Work out the finished part from the listing and answer in its coordinate system (mm). Face numbers are marked on the shaded views. Round coordinates to 2 decimals unless told otherwise and drop trailing zeros. Order: outer loops, then holes, each group sorted by start corner. A loop starts at its lowest first (then second) coordinate and runs counter-clockwise, first axis right, second up. Notation, with made-up numbers: (-37, -39) -> (-26, -39) arc R25 cw to (-26, -13) -> close; hole circle Ø9 at (85, 26). An arc over 180 degrees is marked (long way). Use one line per item in the form item = value.
```python
from build123d import *

# Parameters (mm, degrees)
SKETCH1_W           = 88.9
SKETCH1_H           = 38.1
BOSS_EXTRUDE1_DEPTH = 6.35
CUT_EXTRUDE2_DEPTH  = 6.35


with BuildPart() as part:
    # Sketch1 → Boss-Extrude1 (new body)
    with BuildSketch(Plane.YZ):
        with Locations((44.45, 19.05)):
            Rectangle(SKETCH1_W, SKETCH1_H)
    extrude(amount=BOSS_EXTRUDE1_DEPTH)

    # Sketch2 → Cut-Extrude2 (cut)
    with BuildSketch(Plane.YZ.offset(6.35)):
        with BuildLine():
            Line((31.75, 38.1), (57.15, 38.1))
            ThreePointArc((57.15, 38.1), (44.45, 30.250968343), (31.75, 38.1))
        make_face()
        with BuildLine():
            Line((31.75, 0), (57.15, 0))
            ThreePointArc((57.15, 0), (44.45, 7.326494526), (31.75, 0))
        make_face()
    extrude(amount=-CUT_EXTRUDE2_DEPTH, mode=Mode.SUBTRACT)


solid = part.part
```
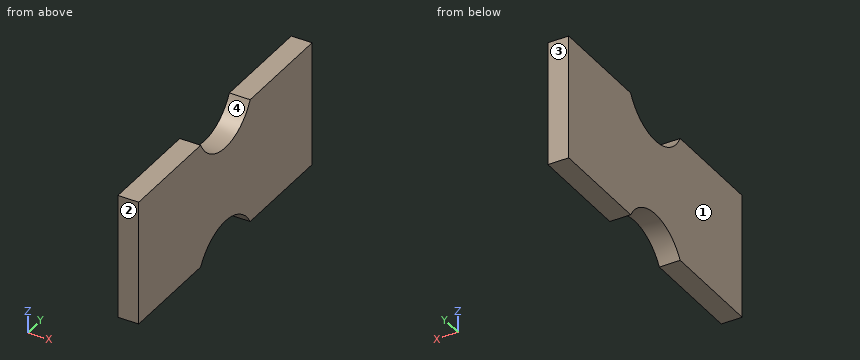
Item 1: The part is cut by section B-B, the plane z = 34.5. Give the vertices of the cut face in (x, y), and give its area (3 significant figures).
Findings:
outline = (0, 0) -> (6.35, 0) -> (6.35, 34.32) -> (0, 34.32) -> close; (0, 54.58) -> (6.35, 54.58) -> (6.35, 88.9) -> (0, 88.9) -> close
area = 436 mm^2
Item 2: The part is cut by section A-A, the plane x = 4.5. Give the vertices of the cut face in (y, z).
Findings:
outline = (0, 0) -> (31.75, 0) arc R14.67 cw to (57.15, 0) -> (88.9, 0) -> (88.9, 38.1) -> (57.15, 38.1) arc R14.2 cw to (31.75, 38.1) -> (0, 38.1) -> close
Item 3: The part is cut by section C-C, the plane y = 33.5. Give the vertices of the cut face in (x, z).
Findings:
outline = (0, 2.42) -> (6.35, 2.42) -> (6.35, 35.41) -> (0, 35.41) -> close
Item 4: Determine the mould class of the marked faces 1, 2, 3 and 4 for opening direction Y: released by +Y, released by -Y, zero draft, split by the parting line, or undercut.
Findings:
face_1 = zero draft
face_2 = released by -Y
face_3 = released by +Y
face_4 = undercut
Item 5: Consider line 1 along Y through (x, z) = (3.5, 5); line 2 along Y through (x, z) = (6.25, 36.5); line 3 along Z through (x, y) = (2.75, 47.5). Determine where each line is inside the solid, lowest interval first.
Findings:
line_1 = 0 to 36.52, 52.38 to 88.9
line_2 = 0 to 32.69, 56.21 to 88.9
line_3 = 7.01 to 30.58
